Study the drawing (mm; zero at the part's minimum x, y, z) and answer. A direction names the side the tool comes from. Round coordinates to 2 decimals unless told otherwise and drop trailing zeros. Write each loop counter-clockwise with the first axis right and the second up, starting at its lowest first coordinate (ties: lowest second). Pieces come first, ordered by that corner, then holes. Notation, with made-up numbers: (46.25, 70.25) - (88.25, 70.25) arc R22 cw to (88.25, 78.25) - close; hole circle Ø5 at (-9, 25.25). An arc over 180 degrees is marked (long way). Use one line per item in the form item = value. Start each with the question number.
1) The part is cut by section B-B, the plane x = 12.5. Give the vertices of the cut face in (y, z) (1 decimal), plus the area to 3 significant figures.
2) For the marked faces 1, 2 and 3, determine the directions among +Z, -Z, +X, -X, +Y, -Y from which every point of the face is accessible in a straight line to the end or side of a thin tool.
3) The part is cut by section C-C, the plane x = 18. Give the vertices of the cut face in (y, z).
4) The part is cut by section D-D, the plane z = 1.25. Give the vertices of the cut face in (x, y), plus the area to 3 significant figures.
5) Consider line 1 along X through (y, z) = (11.5, 8.75); line 2 along Z through (x, y) = (8.25, 14); line 3 along Z through (x, y) = (3.5, 36). Determine where each line is inside the solid, lowest interval first. Write a range as from..to.
6) Each of these flat-tipped pins is pushed along its axis until it touches: pin 1 (1.9 mm diameter, centred on x = 3, y = 37, fed in from -Z); pin 2 (2 mm diameter, centred on x = 7.5, y = 30, fed in from -Z); pin 3 (1.1 mm diameter, centred on y = 37, z = 8.5, fed in from +X); pin 4 (5 mm diameter, centred on x = 3, y = 12.5, fed in from +Z). Where does it stop, or does it pass through?
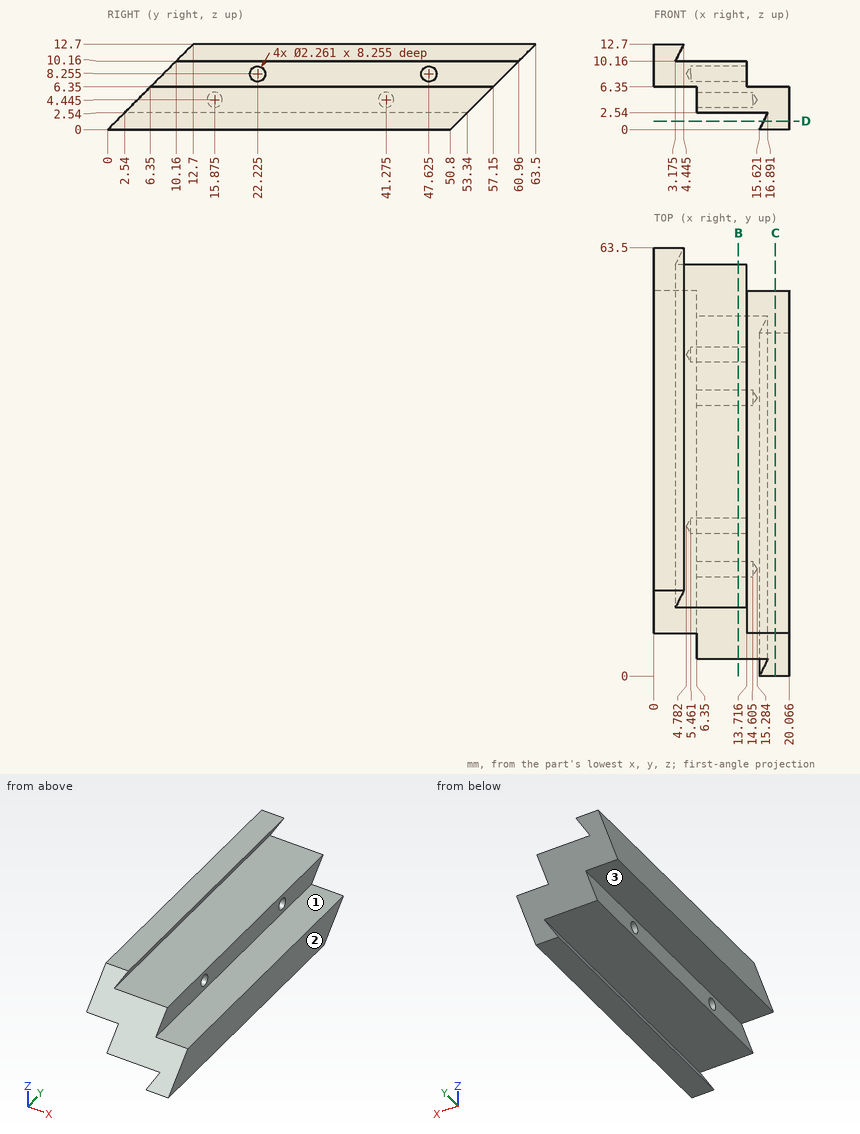
Geometry results:
q1.outline = (2.5, 2.5) - (53.3, 2.5) - (61, 10.2) - (10.2, 10.2) - close; hole circle Ø2.3 at (15.9, 4.4); hole circle Ø2.3 at (22.2, 8.3); hole circle Ø2.3 at (41.3, 4.4); hole circle Ø2.3 at (47.6, 8.3)
q1.area = 371 mm2
q2.face_1 = +Z, +X, +Y, -Y
q2.face_2 = +Z, -Z, +X, +Y, -Y
q2.face_3 = -Z, -X, +Y, -Y
q3.outline = (0, 0) - (50.8, 0) - (57.15, 6.35) - (6.35, 6.35) - close
q4.outline = (16.25, 1.25) - (20.07, 1.25) - (20.07, 52.05) - (16.25, 52.05) - close
q4.area = 194 mm2
q5.line_1 = 0..13.72
q5.line_2 = 2.54..10.16
q5.line_3 = 6.35..10.16, 10.81..12.7
q6.pin_1 = 6.35
q6.pin_2 = 2.54
q6.pin_3 = 13.72
q6.pin_4 = 12.7
